```python
from build123d import *

# Parameters (mm, degrees)
SKETCH1_W           = 70
SKETCH1_H           = 50
BOSS_EXTRUDE1_DEPTH = 50
CUT_EXTRUDE1_DEPTH  = 50
CUT_EXTRUDE2_DEPTH  = 50
CUT_EXTRUDE3_DEPTH  = 30
BOSS_EXTRUDE2_DEPTH = 30
CUT_EXTRUDE4_DEPTH  = 54
SKETCH7_W           = 70
SKETCH7_H           = 50
CUT_EXTRUDE5_DEPTH  = 54
SKETCH8_W           = 70
SKETCH8_H           = 49.997172982
CUT_EXTRUDE6_DEPTH  = 54
BOSS_EXTRUDE3_DEPTH = 30


with BuildPart() as part:
    # Sketch1 → Boss-Extrude1 (new body)
    with BuildSketch(Plane.XY):
        with Locations((35, 25)):
            Rectangle(SKETCH1_W, SKETCH1_H)
    extrude(amount=BOSS_EXTRUDE1_DEPTH)

    # Sketch2 → Cut-Extrude1 (cut)
    with BuildSketch(Plane.XY.offset(50)):
        Polygon((0, 30), (20, 30), (50, 50), (0, 50), align=None)
    extrude(amount=-CUT_EXTRUDE1_DEPTH, mode=Mode.SUBTRACT)

    # Sketch3 → Cut-Extrude2 (cut)
    with BuildSketch(Plane(origin=(70, 0, 0), x_dir=(0, 0, -1), z_dir=(1, 0, 0))):
        Polygon((-50, 40), (-20, 40), (-10, 50), (-50, 50), align=None)
    extrude(amount=-CUT_EXTRUDE2_DEPTH, mode=Mode.SUBTRACT)

    # Sketch4 → Cut-Extrude3 (cut)
    with BuildSketch(Plane.XY.offset(50)):
        Polygon((40, 10), (60, 40), (35, 40), (20, 30), (0, 30), (0, 10), align=None)
    extrude(amount=-CUT_EXTRUDE3_DEPTH, mode=Mode.SUBTRACT)

    # Sketch5 → Boss-Extrude2 (add)
    with BuildSketch(Plane(origin=(0, 30, 30), x_dir=(-1, 0, 0), z_dir=(0, -0.707106781, -0.707106781))):
        Polygon((-70, 28.284271247), (-40, -28.284271247), (0, -28.284271247), (0, 0), (-50, 28.284271247), align=None)
    extrude(amount=BOSS_EXTRUDE2_DEPTH)

    # Sketch6 → Cut-Extrude4 (cut)
    with BuildSketch(Plane(origin=(0, 0, 0), x_dir=(-1, 0, 0), z_dir=(0, 0, -1))):
        Polygon((-50, 50), (-20, 30), (0, 30), (0, 60), (-50, 60), align=None)
    extrude(amount=-CUT_EXTRUDE4_DEPTH, mode=Mode.SUBTRACT)

    # Sketch7 → Cut-Extrude5 (cut)
    with BuildSketch(Plane.XZ):
        with Locations((35, 25)):
            Rectangle(SKETCH7_W, SKETCH7_H)
    extrude(amount=CUT_EXTRUDE5_DEPTH, mode=Mode.SUBTRACT)

    # Sketch8 → Cut-Extrude6 (cut)
    with BuildSketch(Plane(origin=(0, 0, 0), x_dir=(-1, 0, 0), z_dir=(0, 0, -1))):
        with Locations((-35, 24.998586491)):
            Rectangle(SKETCH8_W, SKETCH8_H)
    extrude(amount=CUT_EXTRUDE6_DEPTH, mode=Mode.SUBTRACT)

    # Sketch9 → Boss-Extrude3 (add)
    with BuildSketch(Plane(origin=(0, 30, 0), x_dir=(1, 0, 0), z_dir=(0, 1, 0))):
        Polygon((12.5, -20), (0, -20), (0, -30), align=None)
    extrude(amount=-BOSS_EXTRUDE3_DEPTH)


solid = part.part
```
The listing builds one solid part. Answer for the finished solid, in the listing's coordinates (mm). A direction names the side the tool comes from. Give positions to 0.01 mm unless a question says otherwise; leave off trailing zeros. Order: outer loops, then holes, each group sorted by start corner. A loop starts at its lowest first (then second) coordinate and runs counter-clockwise, first axis right, second up. Notation, with made-up numbers: M 5.25,22.25 L 58.25,22.25 A15 cw 58.25,51.25 Z; hole C 62.25,13 d11. An arc over 180 degrees is marked long. Put each result on its own line as item: value. Start each with the question number.
Item 1: The part is cut by section A-A, the plane y = 13. Determine the outline of the cut face in (x, z), and give its area (3 significant figures).
Item 2: Find the intervals of material crossed by line 1 along Y through (x, z) = (12, 30); line 2 along X through (y, z) = (25, 39); line 3 along Z through (x, y) = (15, 21), in increasing order.
Item 3: Which of the six approach directions +Z, -Z, +X, -X, +Y, -Y give full straight-line access (tool end or side, diameter ignored) to faces 1 (the face through (65, 40, 35)), 2 (the face through (54, 31, 42)), 3 (the face through (10, 30, 15))?
Item 4: The part is cut by section D-D, the plane y = 44.5. Determine the outline of the cut face in (x, z), and give its area (3 significant figures).
Item 5: Flat-ended cylindrical pins translate along their axes: P1, Ø8, axis at x = 66, z = 33, coming from the +Y side; P2, Ø6, axis at x = 5.5, z = 22, coming from the +Y side. Find the tip coordinate at first contact, or state that the pin passes through.
Item 6: The part is cut by section B-B, the plane z = 18. Determine the outline of the cut face in (x, y).
Item 7: The part is cut by section C-C, the plane x = 18. Determine the outline of the cut face in (y, z).
Answer key:
1. outline: M 0,0 L 70,0 L 70,50 L 42,50 L 42,47 L 0,47 Z
1. area: 3,370 mm²
2. line 1: y = 0 to 30
2. line 2: x = 50 to 70
2. line 3: z = 0 to 39
3. face 1: +Z, +X, -X, +Y
3. face 2: +Z, -X, +Y
3. face 3: +Z, -Z, -X, +Y
4. outline: M 41.75,0 L 70,0 L 70,15.5 L 41.75,15.5 Z
4. area: 438 mm²
5. P1: stops at y = 40
5. P2: stops at y = 30
6. outline: M 0,0 L 70,0 L 70,42 L 38,42 L 20,30 L 0,30 Z
7. outline: M 0,0 L 30,0 L 30,30 L 10,50 L 0,50 Z
